Model file for the job. Use its own axes, mm. Face numbers are marked on the shaded views. A direction names the side the tool comes from. Round coordinates to 2 decimals unless told otherwise and drop trailing zeros. Order: outer loops, then holes, each group sorted by start corner. A loop starts at its lowest first (then second) coordinate and runs counter-clockwise, first axis right, second up. Notation, with made-up numbers: M 59.25,82.5 L 99.25,82.5 A24 ccw 99.25,119.5 Z; hole C 28.5,-10 d9. An arc over 180 degrees is marked long. Return JSON: item names as keys, results as strings. Group by question number.
Item 1: Which spindle directions (+Z, -Z, +X, -X, +Y, -Y) get a long thin tool onto all of the face, cutting with end or side? Do the marked faces 5, 6, 7, 8 and 9. Say none if no direction does.
Item 2: Probe line 1 along Z through (x, y) = (0, 12.5); line 2 along Y through (x, z) = (19, 0). List the from-to ranges inside material, lowest first.
Item 3: Pull direction Y, two halves, no side cores. Call the marked faces 1, 2, 3 and 4: pulls with the +Y half, pulls with the -Y half, needs draft (parallel to the pull), parting line crosses it, or undercut.
Item 4: Slice it at D-D on x = 19.5. Write the cut outline in (y, z), then the cut area to 3 significant figures.
Item 5: Slice it at B-B on z = 0. Write the cut outline in (x, y), then the cut area to 3 significant figures.
Item 6: Slice it at C-C on y = 0. Write the cut outline in (x, z).
Item 7: Slice it at A-A on x = 0. Give the number of separate pieces and of enclosed holes in the cut face, then the cut area to 3 significant figures.
Item 8: Pin check, flat tips, straight feed: pin 1 Ø3 at (y, z) = (-10, 4) entering from +X; pin 2 Ø2 at (x, y) = (33.5, 1) entering from -Z; pin 3 Ø6 at (x, z) = (14.5, 3) entering from +Y; pin 4 Ø4.5 at (x, z) = (0, 0) entering from +Y. Stop position of each tip, or through.
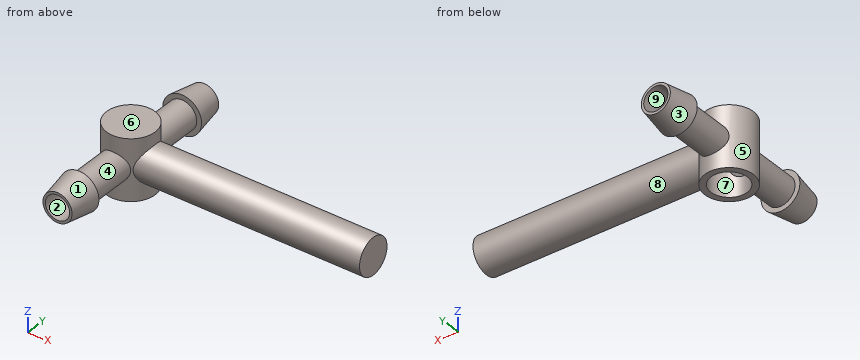
from build123d import *

# Parameters (mm, degrees)
SKETCH1_R           = 5
BOSS_EXTRUDE1_DEPTH = 6.25
SKETCH2_R           = 3
BOSS_EXTRUDE2_DEPTH = 20
SKETCH3_R           = 3.75
BOSS_EXTRUDE3_DEPTH = 50
SKETCH4_R           = 2.5
CUT_EXTRUDE1_DEPTH  = 40
CUT_EXTRUDE2_REACH  = 14.5
SKETCH5_R           = 3.75
SKETCH7_R           = 5
BOSS_EXTRUDE4_DEPTH = 2.5


with BuildPart() as part:
    # Sketch1 → Boss-Extrude1 (new body, symmetric)
    with BuildSketch(Plane.XY):
        Circle(SKETCH1_R)
    extrude(amount=BOSS_EXTRUDE1_DEPTH, both=True)

    # Sketch2 → Boss-Extrude2 (add, symmetric)
    with BuildSketch(Plane(origin=(0, 0, 0), x_dir=(1, 0, 0), z_dir=(0, 1, 0))):
        Circle(SKETCH2_R)
    extrude(amount=BOSS_EXTRUDE2_DEPTH, both=True)

    # Sketch3 → Boss-Extrude3 (add)
    with BuildSketch(Plane(origin=(0, 0, 0), x_dir=(0, 0, -1), z_dir=(1, 0, 0))):
        Circle(SKETCH3_R)
    extrude(amount=BOSS_EXTRUDE3_DEPTH)

    # Sketch4 → Cut-Extrude1 (cut)
    with BuildSketch(Plane.XZ.offset(20)):
        Circle(SKETCH4_R)
    extrude(amount=-CUT_EXTRUDE1_DEPTH, mode=Mode.SUBTRACT)

    # Sketch5 → Cut-Extrude2 (cut, up to next)
    with BuildSketch(Plane.XY.offset(6.25), mode=Mode.PRIVATE) as cut_extrude2_sk1:
        Circle(SKETCH5_R)
    cut_extrude2_tool1 = extrude(cut_extrude2_sk1.sketch, amount=-CUT_EXTRUDE2_REACH, mode=Mode.PRIVATE) & part.part
    add(cut_extrude2_tool1.solids().sort_by_distance((0, 0, 6.25))[0], mode=Mode.SUBTRACT)

    # Sketch6 → Revolve1 (revolve)
    with BuildSketch(Plane.XY):
        Polygon((3, 14), (3, 20), (4, 14), align=None)
        Polygon((3, -20), (4, -14), (3, -14), align=None)
    revolve(axis=Axis((0, 20, 0), (0, -1, 0)))

    # Sketch7 → Boss-Extrude4 (add)
    with BuildSketch(Plane.XY.offset(6.25)):
        Circle(SKETCH7_R)
    extrude(amount=-BOSS_EXTRUDE4_DEPTH)


solid = part.part
Output values:
{
 "1": {"face 5": "none", "face 6": "+Z, +X, -X, +Y, -Y", "face 7": "-Z", "face 8": "+X", "face 9": "+Y, -Y"},
 "2": {"line 1": "-3 to -2.5, 2.5 to 3", "line 2": "-3.75 to 3.75"},
 "3": {"face 1": "pulls with the -Y half", "face 2": "needs draft", "face 3": "pulls with the +Y half", "face 4": "undercut"},
 "4": {"outline": "C 0,0 d7.5", "area": "44.2 mm²"},
 "5": {"outline": "M -4,-14 L -3,-20 L -2.5,-20 L -2.5,-2.8 A3.75 cw -2.5,2.8 L -2.5,20 L -3,20 L -4,14 L -3,14 L -3,4 A5 ccw -3,-4 L -3,-14 Z; M 2.5,-20 L 3,-20 L 4,-14 L 3,-14 L 3,-4 A5 ccw 3.31,-3.75 L 50,-3.75 L 50,3.75 L 3.31,3.75 A5 ccw 3,4 L 3,14 L 4,14 L 3,20 L 2.5,20 L 2.5,2.8 A3.75 cw 2.5,-2.8 Z", "area": "406 mm²"},
 "6": {"outline": "M -5,-6.25 L -3.75,-6.25 L -3.75,3.75 L 3.75,3.75 L 3.75,-6.25 L 5,-6.25 L 5,-3.75 L 50,-3.75 L 50,3.75 L 5,3.75 L 5,6.25 L -5,6.25 Z"},
 "7": {"separate pieces": "3", "enclosed holes": "0", "area": "79.5 mm²"},
 "8": {"pin 1": "x = 1.66", "pin 2": "z = -3.75", "pin 3": "y = 3.75", "pin 4": "through"}
}
